For this review, use the dimensioned drawing (mm, ordinates from the lowest corner) and the shaded views. Give positions to 0.01 mm unless a question says otherwise; leave off trailing zeros. Order: outer loops, then holes, each group sorted by start corner. A loop starts at its lowest first (then second) coordinate and runs counter-clockwise, first axis right, second up.
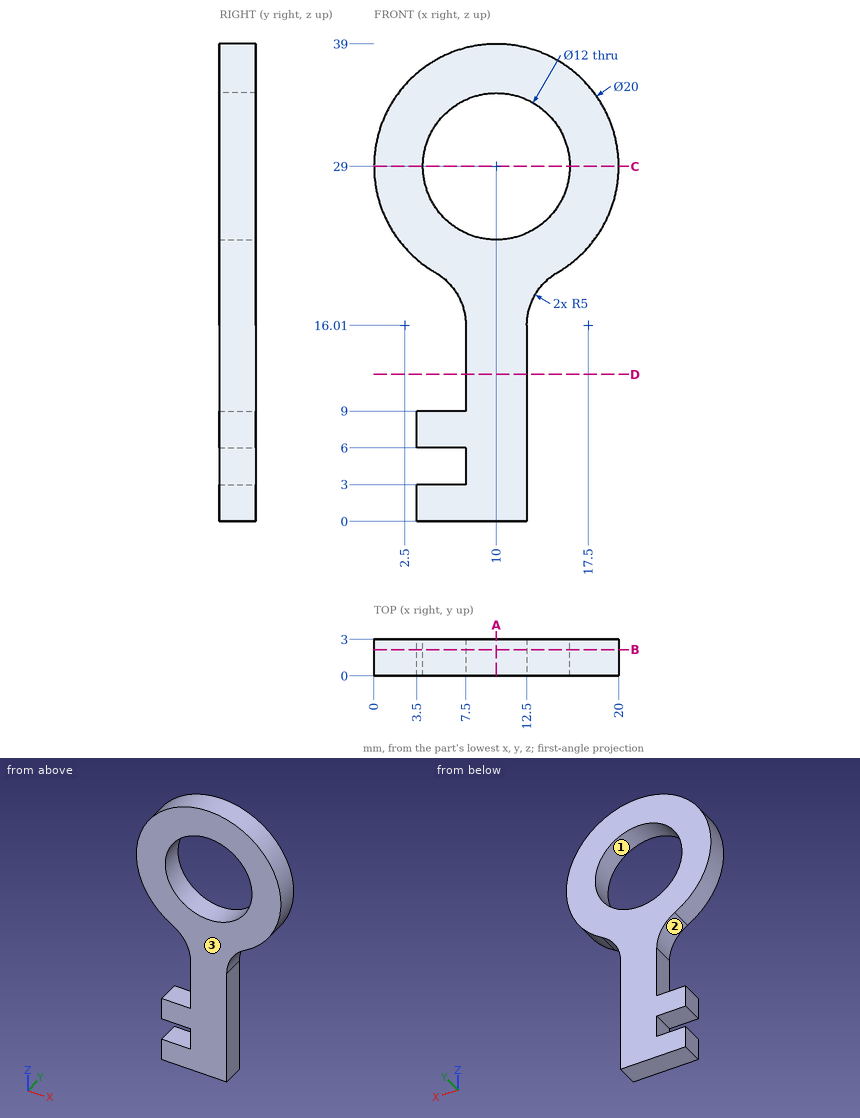
1. Take a section at B-B (y = 2.15). State the section outline as (x, z) points, then the cut area to 3 significant figures.
Recorded:
outline: (3.5, 0) - (12.5, 0) - (12.5, 16.01) arc R5 cw to (15, 20.34) arc R10 ccw (long way) to (5, 20.34) arc R5 cw to (7.5, 16.01) - (7.5, 9) - (3.5, 9) - (3.5, 6) - (7.5, 6) - (7.5, 3) - (3.5, 3) - close; hole circle Ø12 at (10, 29)
area: 324 mm2
2. Take a section at A-A (x = 10). State the section outline as (y, z) points.
Recorded:
outline: (0, 0) - (3, 0) - (3, 23) - (0, 23) - close; (0, 35) - (3, 35) - (3, 39) - (0, 39) - close
3. Take a section at C-C (z = 29). State the section outline as (x, y) points.
Recorded:
outline: (0, 0) - (4, 0) - (4, 3) - (0, 3) - close; (16, 0) - (20, 0) - (20, 3) - (16, 3) - close
4. For line 1 along X through (y, z) = (1.75, 31.5) (1 decimal); line 2 along Z through (x, y) = (11.5, 0.5); line 3 along X through (y, z) = (0.9, 31), list the stretches that pass through material, from the lowest coordinate up.
Recorded:
line 1: x = 0.3 to 4.5, 15.5 to 19.7
line 2: z = 0 to 23.19, 34.81 to 38.89
line 3: x = 0.2 to 4.34, 15.66 to 19.8
5. For pin 1 (0.9 mm diameter, centred on y = 1, z = 13.5, fed in from -X); pin 2 (1 mm diameter, centred on x = 9.5, y = 2, fed in from +Z); pin 3 (1.5 mm diameter, centred on y = 1, z = 8, fed in from -X); pin 4 (1.5 mm diameter, centred on y = 2, z = 12, fed in from +X), all flat-tipped, find the tip position at first contact; note any pin that passes through.
Recorded:
pin 1: stops at x = 7.5
pin 2: stops at z = 39
pin 3: stops at x = 3.5
pin 4: stops at x = 12.5
6. Take a section at D-D (z = 12). State the section outline as (x, y) points.
Recorded:
outline: (7.5, 0) - (12.5, 0) - (12.5, 3) - (7.5, 3) - close
7. Draft analysis for pull direction Z (two halves, no side actions). For the marked faces 1, 2 and 3, state which applies: pulls with the +Z half, pulls with the -Z half, needs draft (parallel to the pull), parting line crosses it, or undercut.
Recorded:
face 1: undercut
face 2: undercut
face 3: needs draft
